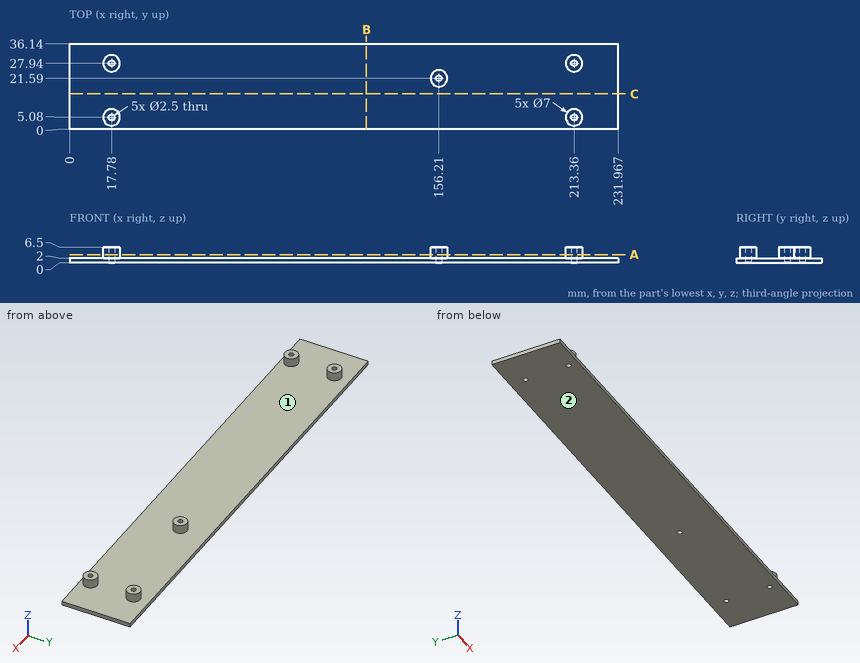
Geometry check sheet. Reference: drawing and pictorial views, mm from the part's lowest x, y, z. Round coordinates to 2 decimals unless told otherwise and drop trailing zeros. Write each loop counter-clockwise with the first axis right and the second up, starting at its lowest first coordinate (ties: lowest second). Pieces come first, ordered by that corner, then holes.
(1) Mould release check, pull along X, two halves, no side actions. Record for the marked faces 1 and 2: pulls with the +X half, pulls with the -X half, needs draft (parallel to the pull), parting line crosses it, or undercut.
Returned:
face 1: undercut
face 2: needs draft
(2) Depth check by flat-ended pin: pin 1 Ø3 at (x, y) = (213.36, 27.94) entering from +Z; pin 2 Ø2 at (x, y) = (213.36, 5.08) entering from -Z; pin 3 Ø2 at (y, z) = (5.5, 4) entering from -X. Enter the tip coordinate at first touch or a pass-through.
Returned:
pin 1: stops at z = 6.5
pin 2: passes through
pin 3: stops at x = 14.28
(3) Section check A-A (z = 3.5). Give the number of separate pieces and of enclosed holes in the cut face, plus the area to 3 significant figures.
Returned:
separate pieces: 5
enclosed holes: 5
area: 168 mm2
(4) Section check C-C (y = 15). Enter the section's corners in (x, z).
Returned:
outline: (0, 0) - (231.97, 0) - (231.97, 2) - (0, 2) - close
(5) Material ranges on line 1 (Y direction, x = 17.78, z = 1.75); line 2 (Y direction, x = 213.36, z = 3); line 3 (X direction, y = 27.94, z = 4.25), recorded low to high.
Returned:
line 1: y = 0 to 3.83, 6.33 to 26.69, 29.19 to 36.14
line 2: y = 1.58 to 3.83, 6.33 to 8.58, 24.44 to 26.69, 29.19 to 31.44
line 3: x = 14.28 to 16.53, 19.03 to 21.28, 209.86 to 212.11, 214.61 to 216.86
(6) Section check B-B (x = 125.5). Enter the section's corners in (y, z).
Returned:
outline: (0, 0) - (36.14, 0) - (36.14, 2) - (0, 2) - close
